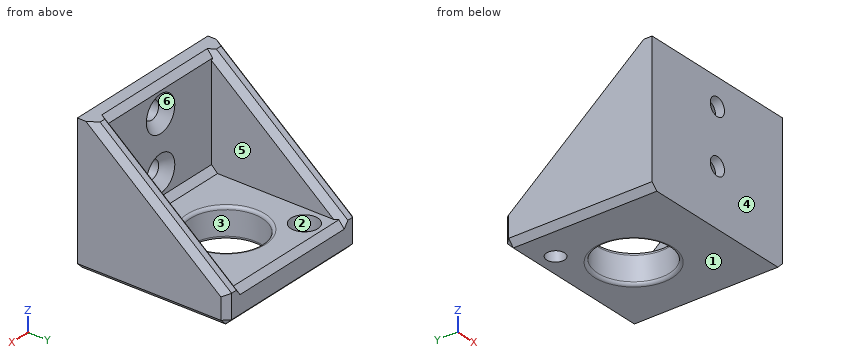
from build123d import *

# Parameters (mm, degrees)
ESBO_O1_W                = 27.5
ESBO_O1_H                = 25
RESSALTO_EXTRUS_O1_DEPTH = 5
ESBO_O2_W                = 27.5
ESBO_O2_H                = 3
RESSALTO_EXTRUS_O2_DEPTH = 18
RESSALTO_EXTRUS_O3_DEPTH = 3
RESSALTO_EXTRUS_O4_DEPTH = 3
ESBO_O5_R                = 1.5
CORTE_EXTRUS_O1_DEPTH    = 5
CHANFRO1_SIZE            = 1.5
CHANFRO2_SIZE            = 1
CHANFRO4_SIZE            = 1
CHANFRO5_SIZE            = 1
ESBO_O6_R                = 6
ESBO_O6_R_2              = 1.5
CORTE_EXTRUS_O2_DEPTH    = 5
FILETE1_R                = 0.5
ESBO_O8_R                = 2.25
CORTE_EXTRUS_O3_DEPTH    = 2.5


with BuildPart() as part:
    # Esboço1 → Ressalto-extrusão1 (new body)
    with BuildSketch(Plane.XY):
        Rectangle(ESBO_O1_W, ESBO_O1_H)
    extrude(amount=RESSALTO_EXTRUS_O1_DEPTH)

    # Esboço2 → Ressalto-extrusão2 (add)
    with BuildSketch(Plane.XY.offset(5)):
        with Locations((0, -11)):
            Rectangle(ESBO_O2_W, ESBO_O2_H)
    extrude(amount=RESSALTO_EXTRUS_O2_DEPTH)

    # Esboço3 → Ressalto-extrusão3 (add)
    with BuildSketch(Plane(origin=(13.75, 0, 0), x_dir=(0, 0, -1), z_dir=(1, 0, 0))):
        Polygon((-5, 12.5), (-23, -9.5), (-5, -9.5), align=None)
    extrude(amount=-RESSALTO_EXTRUS_O3_DEPTH)

    # Esboço4 → Ressalto-extrusão4 (add)
    with BuildSketch(Plane.ZY.offset(13.75)):
        Polygon((5, 12.5), (5, -9.5), (23, -9.5), align=None)
    extrude(amount=-RESSALTO_EXTRUS_O4_DEPTH)

    # Esboço5 → Corte-extrusão1 (cut)
    with BuildSketch(Plane(origin=(0, -9.5, 0), x_dir=(1, 0, 0), z_dir=(0, 1, 0))):
        with Locations(Location((0, -9.5, 0), (0, 0, 270))):
            Circle(ESBO_O5_R)
        with Locations(Location((0, -18.5, 0), (0, 0, 270))):
            Circle(ESBO_O5_R)
    extrude(amount=-CORTE_EXTRUS_O1_DEPTH, mode=Mode.SUBTRACT)

    # Chanfro1
    chanfro1_edges = [part.edges().sort_by_distance(p)[0] for p in [
        (0, -9.5, 8),
        (0, -9.5, 17),
    ]]
    chamfer(chanfro1_edges, length=CHANFRO1_SIZE)

    # Chanfro2
    chanfro2_edges = [part.edges().sort_by_distance(p)[0] for p in [
        (13.75, 1.5, 14),
        (-13.75, 1.5, 14),
        (0, 12.5, 0),
        (13.75, 0, 0),
        (-13.75, 0, 0),
        (-13.75, 12.5, 2.5),
        (13.75, 12.5, 2.5),
    ]]
    chamfer(chanfro2_edges, length=CHANFRO2_SIZE)

    # Chanfro4
    chanfro4_edges = [part.edges().sort_by_distance(p)[0] for p in [
        (10.75, 1.5, 14),
        (-10.75, 1.5, 14),
    ]]
    chamfer(chanfro4_edges, length=CHANFRO4_SIZE)

    # Chanfro5
    chanfro5_edges = [part.edges().sort_by_distance(p)[0] for p in [
        (0, -9.5, 23),
        (0, -9.5, 5),
        (0, 12.5, 5),
    ]]
    chamfer(chanfro5_edges, length=CHANFRO5_SIZE)

    # Esboço6 → Corte-extrusão2 (cut)
    with BuildSketch(Plane.XY.offset(5)):
        with Locations((0, 1.5)):
            Circle(ESBO_O6_R)
        with Locations((-7.571529996, 8.543317004)):
            Circle(ESBO_O6_R_2)
    extrude(amount=-CORTE_EXTRUS_O2_DEPTH, mode=Mode.SUBTRACT)

    # Filete1
    filete1_edges = [part.edges().sort_by_distance(p)[0] for p in [
        (-6, 1.5, 0),
        (-6, 1.5, 5),
    ]]
    fillet(filete1_edges, radius=FILETE1_R)

    # Esboço8 → Corte-extrusão3 (cut)
    with BuildSketch(Plane.XY.offset(5)):
        with Locations((-7.571529996, 8.543317004)):
            Circle(ESBO_O8_R)
    extrude(amount=-CORTE_EXTRUS_O3_DEPTH, mode=Mode.SUBTRACT)


solid = part.part
Geometry: final body of the model. Coordinates: model frame, mm. Face numbers are marked on the shaded views. A direction names the side the tool comes from. Give positions to 0.01 mm unless a question says otherwise; leave off trailing zeros. Write each loop counter-clockwise with the first axis right and the second up, starting at its lowest first coordinate (ties: lowest second). Pieces come first, ordered by that corner, then holes. Notation, with made-up numbers: (88, -37) - (128, -37) arc R27 ccw to (128, -7) - close; hole circle Ø8 at (-32, -32). An arc over 180 degrees is marked (long way). Return JSON: item names as keys, results as strings. Group by question number.
1) Section A-A on x = 0. State how many separate pieces and enclosed holes the cut face has, plus the area to 3 significant figures.
2) First-contact query: P1, Ø8, axis at x = -2, z = 16, coming from the +Y side; P2, Ø7, axis at x = -7.57, y = 8.54, coming from the +Z side; P3, Ø14, axis at x = 0, y = 1.5, coming from the +Z side; P4, Ø1.8, axis at x = -7.57, y = 8.54, coming from the -Z side. Flat tips, straight axial feed; report the tip coordinate or a pass-through.
3) Line query: line 1 (X direction, y = -1.25, z = 11); line 2 (X direction, y = -11.4, z = 18.5); line 3 (Y direction, x = -7.5, z = 16). Output: solid intervals per line, ascending.
4) Section B-B on z = 9.5. Return the cut outline in (x, y), plus the area to 3 significant figures.
5) Mould query, pull axis Y, two halves, no side actions, for the marked faces 1, 2, 3 and 4. Classes: released by +Y, released by -Y, zero draft, split by the parting line, or undercut.
6) Set-up query: the marked faces 5 and 6. Return all of +Z, -Z, +X, -X, +Y, -Y with unobstructed straight access to the full face (end or side cutting, diameter ignored); none if empty.
7) Section D-D on y = 1.5. Return the cut outline in (x, z).
8) Section C-C on x = 9. Return the cut outline in (y, z).
Filled in:
{
 "1": {"separate pieces": "4", "enclosed holes": "0", "area": "95.3 mm^2"},
 "2": {"P1": "stops at y = -9.5", "P2": "stops at z = 8.14", "P3": "stops at z = 5", "P4": "passes through"},
 "3": {"line 1": "x = -13.75 to -10.75, 10.75 to 13.75", "line 2": "x = -13.75 to -1.5, 1.5 to 13.75", "line 3": "y = -12.5 to -9.5"},
 "4": {"outline": "(-13.75, -12.5) - (-1.5, -12.5) - (-1.5, -11) - (-3, -9.5) - (-10.75, -9.5) - (-10.75, 5.42) - (-11.75, 7) - (-12.75, 7) - (-13.75, 5.42) - close; (1.5, -12.5) - (13.75, -12.5) - (13.75, 5.42) - (12.75, 7) - (11.75, 7) - (10.75, 5.42) - (10.75, -9.5) - (3, -9.5) - (1.5, -11) - close", "area": "167 mm^2"},
 "5": {"face 1": "zero draft", "face 2": "undercut", "face 3": "undercut", "face 4": "released by -Y"},
 "6": {"face 5": "+Z, +Y", "face 6": "+Y"},
 "7": {"outline": "(-13.75, 1) - (-12.75, 0) - (-6.5, 0) arc R0.5 ccw to (-6, 0.5) - (-6, 4.5) arc R0.5 ccw to (-6.5, 5) - (-10.75, 5) - (-10.75, 12.71) - (-11.75, 14) - (-12.75, 14) - (-13.75, 12.71) - close; (6, 0.5) arc R0.5 ccw to (6.5, 0) - (12.75, 0) - (13.75, 1) - (13.75, 12.71) - (12.75, 14) - (11.75, 14) - (10.75, 12.71) - (10.75, 5) - (6.5, 5) arc R0.5 ccw to (6, 4.5) - close"},
 "8": {"outline": "(-12.5, 0) - (11.5, 0) - (12.5, 1) - (12.5, 4) - (11.5, 5) - (-8.5, 5) - (-9.5, 6) - (-9.5, 22) - (-10.5, 23) - (-12.5, 23) - close"}
}
